Can you work these out from the model? Positions are in its coordinate system, mm. A direction names the side the tool comes from. Coordinates: 2 decimals unless noted, no trailing zeros. Order: outer loops, then holes, each group sorted by start corner. A loop starts at its lowest first (then second) coordinate and runs counter-clockwise, first axis right, second up. Notation, with made-up numbers: (59, 55.5) - (107, 55.5) arc R31 ccw to (107, 80.5) - close; hole circle Ø10 at (56, 84). An arc over 180 degrees is marked (long way). Return JSON: item names as keys, results as strings. Group by question number.
1) If I drill on line 1 along Z through (x, y) = (0.9, 4); line 2 along Z through (x, y) = (0.75, -3.25); line 3 along Z through (x, y) = (0.95, -3.75), over which ranges is the centre line in solid material (lowest first)?
2) Which directions (+Z, -Z, +X, -X, +Y, -Y) give clear straight access to the entire face, cutting with the end or side of a thin tool? Please do faces 4 (the face through (1.5, -6, 3)), 5 (the face through (1, -0.5, -9)), 6 (the face through (1, -10, 15)).
3) If we mould it in two halves opening along Y, with no side actions, what happens to faces 1 (the face through (0.74, -4.93, 9.46)), 2 (the face through (0.74, 4.62, -2.55)), 3 (the face through (0.74, -13.07, 20.75))? For each: pulls with the +Y half, pulls with the -Y half, needs draft (parallel to the pull), parting line crosses it, or undercut.
4) For pin 1 Ø4 at (y, z) = (-13, 9.75) entering from +X, with a flat end and sliding along its axis, tell me the tip position at first contact or that it passes through.
5) Imagine slicing it at D-D (y = -3.25). Write out the boundary of the cut face in (x, z), and give its area (3 significant figures).
6) Imagine slicing it at B-B (x = 1.25). Write out the boundary of the cut face in (y, z), and give its area (3 significant figures).
7) Imagine slicing it at A-A (y = -13). Write out the boundary of the cut face in (x, z), and give its area (3 significant figures).
8) Imagine slicing it at C-C (z = 17). Write out the boundary of the cut face in (x, y).
Autodesk Inventor part; units mm, degrees
ref_plane "YZ Plane" through (0, 0, 0) normal (1, 0, 0) x (0, 1, 0)
ref_plane "XZ Plane" through (0, 0, 0) normal (0, 1, 0) x (-1, 0, 0)
ref_plane "XY Plane" through (0, 0, 0) normal (0, 0, 1) x (1, 0, 0)
sketch "スケッチ1" plane through (0, 0, 0) normal (1, 0, 0) x (0, 1, 0)
  line L0 (7, 0) -> (-7, 0)
  line L1 (-7, 0) -> (-7, -6.75)
  line L2 (-7, -6.75) -> (7, -6.75)
  line L3 (7, -6.75) -> (7, 0)
  circle A0 centre (4, -3.75) radius 3
  circle A1 centre (-4, -3.75) radius 3
  line L4 (7, -0.75) -> (-7, -0.75)
  line L5 (-7, 0) -> (-7, 6.75)
  line L6 (-7, 6.75) -> (7, 6.75)
  line L7 (7, 6.75) -> (7, 0)
  circle A2 centre (4, 3.75) radius 3
  circle A3 centre (-4, 3.75) radius 3
  line L8 (7, 0.75) -> (-7, 0.75)
  circle A4 centre (4, -3.75) radius 1.35
  circle A5 centre (-4, -3.75) radius 1.35
  circle A6 centre (-4, 3.75) radius 1.35
  circle A7 centre (4, 3.75) radius 1.35
  line L9 (0, -21.85) -> (0, 27.85)
  line L10 (-10, 20.75) -> (-16, 20.75)
  line L11 (-16, 20.75) -> (-16, 3.75)
  line L12 (-16, 3.75) -> (-10, 3.75)
  line L13 (-10, 3.75) -> (-10, 20.75)
  circle A8 centre (-13, 17.75) radius 1.6
  circle A9 centre (-13, 9.75) radius 1.6
  circle A10 centre (-13, 17.75) radius 3
  line L14 (-7, -6.75) -> (-0.5, -6.75)
  line L15 (-0.5, -6.75) -> (-0.5, -14.75)
  line L16 (-0.5, -14.75) -> (-7, -14.75)
  line L17 (-7, -14.75) -> (-7, -6.75)
  circle A11 centre (-4, -11.25) radius 1.6
  circle A12 centre (-4, -11.25) radius 3.5
  line L18 (-16, 3.75) -> (-7, 0)
  line L19 (0, 6.75) -> (-10, 12.25)
  point P0 (0, 0)
  point P1 (0, 0)
  point P2 (-4.1535, 3.75)
  point P3 (7, -3.75)
  point P4 (7, 3.75)
  point P5 (-7, 3.75)
  point P6 (-7, -3.75)
  point P7 (4, 6.75)
  point P8 (-4, 6.75)
  point P9 (-16, 17.75)
  point P10 (-7, 6.75)
  point P11 (-5.3457, 6.75)
  point P12 (-10, 17.75)
  point P13 (2.4272, 6.3046)
  point P14 (-7, 3.75)
  point P15 (-7, -13.0528)
  point P16 (-0.5, -11.25)
  point P17 (4, -6.75)
  dimension "d0" = 14
  dimension "d1" = 6
  dimension "d2" = 6
  dimension "d3" = 0.75
  dimension "d5" = 2.7
  dimension "d12" = 6
  dimension "d13" = 3.2
  dimension "d14" = 3.2
  dimension "d15" = 3
  dimension "d16" = 8
  dimension "d17" = 3
  dimension "d19" = 3.2
  dimension "d20" = 8
  dimension "d21" = 3.5
  dimension "d22" = 3
extrude "プレート1" add sketch "スケッチ1" along normal blind 1.5 contours L3 L4 L9 L0 | L0 L9 L8 L7 | L9 L4 L1 L0 | L0 L5 L8 L9 | L3 A0 L4 | L8 A2 L7 | L18 L12 L13 L19 L6 L5 | L9 L2 A1 L4 | L4 A0 L2 L9 | L9 L6 A2 L8 | L8 A3 L6 L9 | A0 | A2 | L4 A1 L1 | L5 A3 L8 | L11 A10 L13 L12 | A1 | A3 | A1 L2 L1 | L5 L6 A3 | A10 | L15 A12 L17 L2 | A12 L17 picked at (-6.5333, -11.25)
equation "\"d17\" = 0.5 * d10"
equation "\"d6\" = Thickness"
equation "\"BendRadius\" = Thickness"
equation "\"BendReliefWidth\" = Thickness"
equation "\"BendReliefDepth\" = 0.5 * Thickness"
equation "\"CornerReliefSize\" = 4 * Thickness"
equation "\"MinimumRemnant\" = 2 * Thickness"
equation "\"TransitionRadius\" = BendRadius"
equation "\"JacobiRadiusSize\" = BendRadius"
equation "\"GapSize\" = Thickness"
properties part number "fork_outside" material "アルミニウム 6061"
Calculated:
{
 "1": {"line 1": "-6.75 to -5.1, -2.4 to 2.4, 5.1 to 6.75", "line 2": "-14.67 to -12.66, -9.84 to -4.87, -2.63 to 2.63, 4.87 to 8.54", "line 3": "-14.74 to -12.83, -9.67 to -5.08, -2.42 to 2.42, 5.08 to 8.81"},
 "2": {"face 4": "+Z, -Z, +X, +Y, -Y", "face 5": "-Z, +X, -X, +Y", "face 6": "+Z, +X, -X, +Y"},
 "3": {"face 1": "pulls with the +Y half", "face 2": "undercut", "face 3": "parting line crosses it"},
 "4": {"pin 1": "x = 1.5"},
 "5": {"outline": "(0, -14.67) - (1.5, -14.67) - (1.5, -12.66) - (0, -12.66) - close; (0, -9.84) - (1.5, -9.84) - (1.5, -4.87) - (0, -4.87) - close; (0, -2.63) - (1.5, -2.63) - (1.5, 2.63) - (0, 2.63) - close; (0, 4.87) - (1.5, 4.87) - (1.5, 8.54) - (0, 8.54) - close", "area": "23.8 mm2"},
 "6": {"outline": "(-16, 3.75) - (-7, 0) - (-7, -13.05) arc R3.5 ccw to (-0.5, -11.25) - (-0.5, -6.75) - (4, -6.75) arc R3 ccw to (7, -3.75) - (7, 3.75) arc R3 ccw to (4, 6.75) - (0, 6.75) - (-10, 12.25) - (-10, 17.75) arc R3 ccw to (-16, 17.75) - close; hole circle Ø3.2 at (-13, 9.75); hole circle Ø3.2 at (-13, 17.75); hole circle Ø3.2 at (-4, -11.25); hole circle Ø2.7 at (-4, -3.75); hole circle Ø2.7 at (-4, 3.75); hole circle Ø2.7 at (4, -3.75); hole circle Ø2.7 at (4, 3.75)", "area": "338 mm2"},
 "7": {"outline": "(0, 2.5) - (1.5, 2.5) - (1.5, 8.15) - (0, 8.15) - close; (0, 11.35) - (1.5, 11.35) - (1.5, 16.15) - (0, 16.15) - close; (0, 19.35) - (1.5, 19.35) - (1.5, 20.75) - (0, 20.75) - close", "area": "17.8 mm2"},
 "8": {"outline": "(0, -16) - (1.5, -16) - (1.5, -14.41) - (0, -14.41) - close; (0, -11.59) - (1.5, -11.59) - (1.5, -10) - (0, -10) - close"}
}
